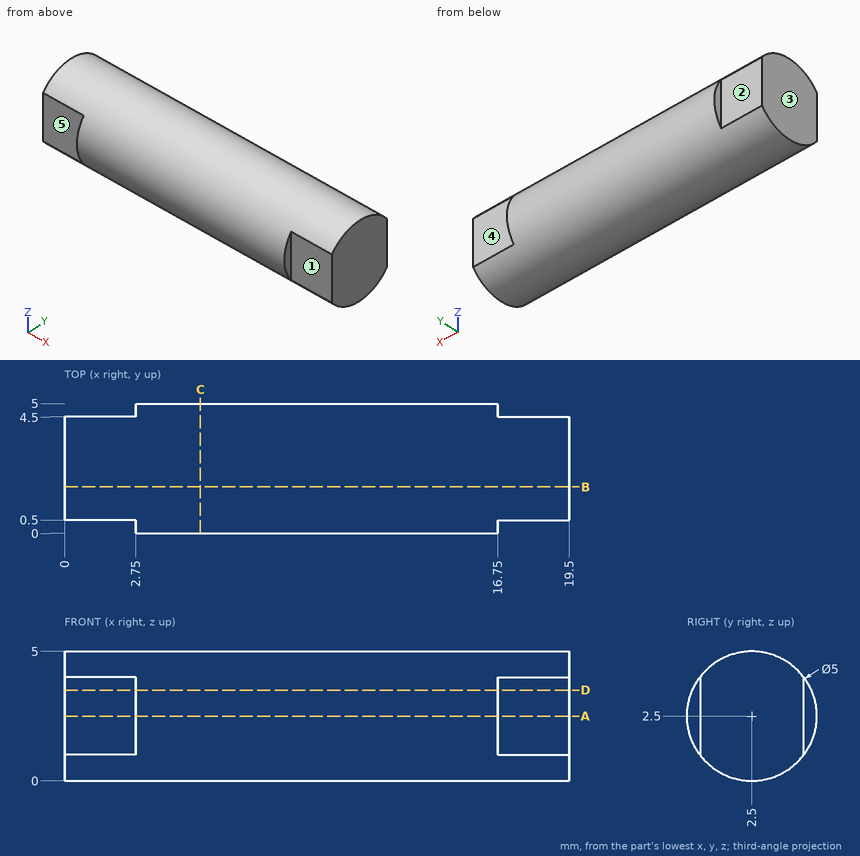
Geometry check sheet. Reference: drawing and pictorial views, mm from the part's lowest x, y, z. A direction names the side the tool comes from. Round coordinates to 2 decimals unless told otherwise and drop trailing zeros. Write each loop counter-clockwise with the first axis right and the second up, starting at its lowest first coordinate (ties: lowest second). Pieces come first, ordered by that corner, then holes.
1. Section check C-C on x = 5.25. Enter the section's corners in (y, z), plus the area to 3 significant figures.
2. Scan lines: L1, parallel to Y at x = 8, z = 0.5; L2, parallel to X at y = 0.4, z = 3.2; L3, parallel to Y at x = 8, z = 2.6. Record each from-to range of solid material in increasing order.
3. Section check B-B on y = 1.8. Enter the section's corners in (x, z).
4. Section check A-A on z = 2.5. Enter the section's corners in (x, y), plus the area to 3 significant figures.
5. Gauge pin test, flat ends, axial feed: P1, Ø0.8, axis at x = 1.5, z = 3, coming from the -Y side; P2, Ø1.4, axis at x = 17.5, z = 2, coming from the +Y side. Record the tip position at first contact, or that the pin passes through.
6. Access from +Z, -Z, +X, -X, +Y, -Y to the whole of each face (thin tool, end or side, straight path). Record for the marked faces 1, 2, 3, 4 and 5.
7. Section check D-D on z = 3.5. Enter the section's corners in (x, y), plus the area to 3 significant figures.
Answer:
1. outline: circle Ø5 at (2.5, 2.5)
1. area: 19.6 mm2
2. L1: y = 1 to 4
2. L2: x = 2.75 to 16.75
2. L3: y = 0 to 5
3. outline: (0, 0.1) - (19.5, 0.1) - (19.5, 4.9) - (0, 4.9) - close
4. outline: (0, 0.5) - (2.75, 0.5) - (2.75, 0) - (16.75, 0) - (16.75, 0.5) - (19.5, 0.5) - (19.5, 4.5) - (16.75, 4.5) - (16.75, 5) - (2.75, 5) - (2.75, 4.5) - (0, 4.5) - close
4. area: 92.0 mm2
5. P1: stops at y = 0.5
5. P2: stops at y = 4.5
6. face 1: +Z, -Z, +X, -Y
6. face 2: +Z, -Z, -X, +Y
6. face 3: +Z, -Z, -X, +Y, -Y
6. face 4: +Z, -Z, +X, +Y
6. face 5: +Z, -Z, -X, -Y
7. outline: (0, 0.5) - (2.75, 0.5) - (2.75, 0.21) - (16.75, 0.21) - (16.75, 0.5) - (19.5, 0.5) - (19.5, 4.5) - (16.75, 4.5) - (16.75, 4.79) - (2.75, 4.79) - (2.75, 4.5) - (0, 4.5) - close
7. area: 86.2 mm2
